Source: CAD feature listing. Evaluate the final solid. Frame: model axes, mm. Face numbers are marked on the shaded views. A direction names the side the tool comes from. Give positions to 0.01 mm unless a question says otherwise; leave off trailing zeros. Loops run counter-clockwise (first coordinate to the right, second up) from the corner with the lowest first, then second, coordinate; pieces in that order, holes last.
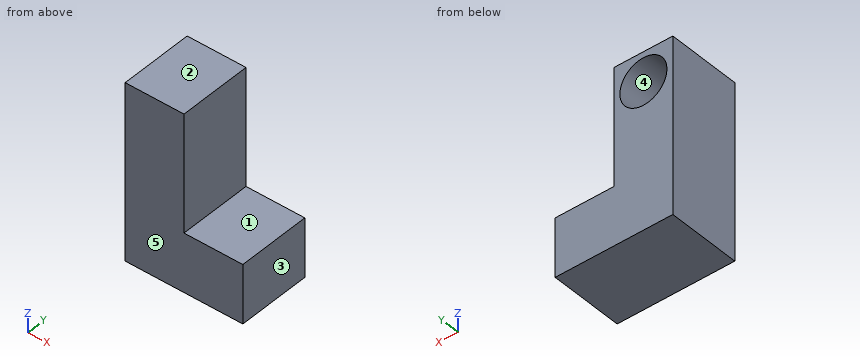
from build123d import *

# Parameters (mm, degrees)
F0_W     = 20
F0_H     = 25
F1_DEPTH = 60
F2_DEPTH = 20
F4_START = -5
F3_R     = 8
F4_DEPTH = 20


with BuildPart() as f1:
    # F0 (on Top) → F1 (new body)
    with BuildSketch(Plane.XY):
        with Locations((-10, 0)):
            Rectangle(F0_W, F0_H)
    extrude(amount=F1_DEPTH)

    # F0 (on Top) → F2 (join)
    with BuildSketch(Plane.XY):
        with Locations((10, 0)):
            Rectangle(F0_W, F0_H)
    extrude(amount=F2_DEPTH)

    # F3 (on face) → F4 (cut)
    with BuildSketch(Plane.XZ.offset(12.5).offset(F4_START)):
        with Locations((-10, 50)):
            Circle(F3_R)
    extrude(amount=-F4_DEPTH, mode=Mode.SUBTRACT)


solid = f1.part
1) Cut plane D-D (z = 39.5). Return loops of the section in (x, y), and give its area (3 significant figures).
Checks:
outline: (-20, -12.5) - (0, -12.5) - (0, 12.5) - (-20, 12.5) - close
area: 500 mm2
2) Cut plane A-A (y = -3.75). Return loops of the section in (x, z).
Checks:
outline: (-20, 0) - (20, 0) - (20, 20) - (0, 20) - (0, 60) - (-20, 60) - close; hole circle Ø16 at (-10, 50)
3) Pull-direction query (X, two-part tool) for the marked faces 3, 4 and 5; classes: released by +X, released by -X, zero draft, split by the parting line, or undercut.
Checks:
face 3: released by +X
face 4: undercut
face 5: zero draft
4) Cut plane B-B (x = -10). Return loops of the section in (y, z).
Checks:
outline: (-12.5, 0) - (12.5, 0) - (12.5, 42) - (-7.5, 42) - (-7.5, 58) - (12.5, 58) - (12.5, 60) - (-12.5, 60) - close
5) Reachability of the marked faces 1 and 2 from +Z, -Z, +X, -X, +Y, -Y: full face, straight path, thin tool, end or side. Return the list, or none.
Checks:
face 1: +Z, +X, +Y, -Y
face 2: +Z, +X, -X, +Y, -Y
6) Contact query for flat-ended pins moving along their axis: P1, Ø8, axis at x = -8, z = 47.5, coming from the +Y side; P2, Ø2, axis at y = 5.5, z = 52.5, coming from the +X side; P3, Ø2, axis at x = 13, y = 7, coming from the -Z side. Output: stop coordinate, or through.
Checks:
P1: stops at y = -7.5
P2: stops at x = 0
P3: stops at z = 0
7) Ray query, probe 1 along Z at (x, y) = (-10, 6.25); probe 2 along Z at (x, y) = (15, -0.75); probe 3 along X at (y, z) = (8.5, 39.5). Return the intervals inside material, ascending.
Checks:
probe 1: z = 0 to 42, 58 to 60
probe 2: z = 0 to 20
probe 3: x = -20 to 0
8) Cut plane C-C (z = 50). Return loops of the section in (x, y).
Checks:
outline: (-20, -12.5) - (0, -12.5) - (0, 12.5) - (-2, 12.5) - (-2, -7.5) - (-18, -7.5) - (-18, 12.5) - (-20, 12.5) - close
